from build123d import *

# Parameters (mm, degrees)
F0_W     = 50.8
F0_H     = 50.8
F1_DEPTH = 50.8
F3_DEPTH = 50.801
F7_DEPTH = 50.801
F9_DEPTH = 50.801
F11_R    = 1.5875


with BuildPart() as f1:
    # F0 (on Front) → F1 (new body)
    with BuildSketch(Plane.XZ):
        with Locations((25.4, 25.4)):
            Rectangle(F0_W, F0_H)
    extrude(amount=F1_DEPTH)

    # F2 (on face) → F3 (cut, through all)
    with BuildSketch(Plane.YZ.offset(50.8)):
        with BuildLine():
            Line((0, 27.305), (0, 43.815))
            ThreePointArc((0, 43.815), (-0.9299359697, 41.5699359697), (-3.175, 40.64))
            Line((-3.175, 40.64), (-37.465, 40.64))
            ThreePointArc((-37.465, 40.64), (-39.7100640303, 39.7100640303), (-40.64, 37.465))
            Line((-40.64, 37.465), (-40.64, 33.655))
            ThreePointArc((-40.64, 33.655), (-39.7100640303, 31.4099359697), (-37.465, 30.48))
            Line((-37.465, 30.48), (-3.175, 30.48))
            ThreePointArc((-3.175, 30.48), (-0.9299359697, 29.5500640303), (0, 27.305))
        make_face()
        with BuildLine():
            ThreePointArc((-47.625, 20.32), (-49.8700640303, 21.2499359697), (-50.8, 23.495))
            Line((-50.8, 23.495), (-50.8, 6.985))
            ThreePointArc((-50.8, 6.985), (-49.8700640303, 9.2300640303), (-47.625, 10.16))
            Line((-47.625, 10.16), (-13.335, 10.16))
            ThreePointArc((-13.335, 10.16), (-11.0899359697, 11.0899359697), (-10.16, 13.335))
            Line((-10.16, 13.335), (-10.16, 17.145))
            ThreePointArc((-10.16, 17.145), (-11.0899359697, 19.3900640303), (-13.335, 20.32))
            Line((-13.335, 20.32), (-47.625, 20.32))
        make_face()
        with BuildLine():
            Line((0, 50.8), (-3.175, 50.8))
            ThreePointArc((-3.175, 50.8), (-0.9299359697, 49.8700640303), (0, 47.625))
            Line((0, 47.625), (0, 50.8))
        make_face()
        with BuildLine():
            ThreePointArc((-50.8, 47.625), (-49.8700640303, 49.8700640303), (-47.625, 50.8))
            Line((-47.625, 50.8), (-50.8, 50.8))
            Line((-50.8, 50.8), (-50.8, 47.625))
        make_face()
        with BuildLine():
            Line((0, 0), (0, 3.175))
            ThreePointArc((0, 3.175), (-0.9299359697, 0.9299359697), (-3.175, 0))
            Line((-3.175, 0), (0, 0))
        make_face()
        with BuildLine():
            ThreePointArc((-47.625, 0), (-49.8700640303, 0.9299359697), (-50.8, 3.175))
            Line((-50.8, 3.175), (-50.8, 0))
            Line((-50.8, 0), (-47.625, 0))
        make_face()
    extrude(amount=-F3_DEPTH, mode=Mode.SUBTRACT)

    # F6 (on offset) → F7 (cut, through all)
    with BuildSketch(Plane.XZ.offset(50.8)):
        with BuildLine():
            ThreePointArc((3.175, 40.64), (0.9299359697, 41.5699359697), (0, 43.815))
            Line((0, 43.815), (0, 17.145))
            ThreePointArc((0, 17.145), (0.9299359697, 19.3900640303), (3.175, 20.32))
            Line((3.175, 20.32), (6.985, 20.32))
            ThreePointArc((6.985, 20.32), (9.2300640303, 19.3900640303), (10.16, 17.145))
            Line((10.16, 17.145), (10.16, 13.335))
            ThreePointArc((10.16, 13.335), (11.0899359697, 11.0899359697), (13.335, 10.16))
            Line((13.335, 10.16), (17.145, 10.16))
            ThreePointArc((17.145, 10.16), (19.3900640303, 11.0899359697), (20.32, 13.335))
            Line((20.32, 13.335), (20.32, 37.465))
            ThreePointArc((20.32, 37.465), (19.3900640303, 39.7100640303), (17.145, 40.64))
            Line((17.145, 40.64), (3.175, 40.64))
        make_face()
        with BuildLine():
            Line((50.8, 50.8), (47.625, 50.8))
            ThreePointArc((47.625, 50.8), (49.8700640303, 49.8700640303), (50.8, 47.625))
            Line((50.8, 47.625), (50.8, 50.8))
        make_face()
        with BuildLine():
            Line((50.8, 0), (50.8, 43.815))
            ThreePointArc((50.8, 43.815), (49.8700640303, 41.5699359697), (47.625, 40.64))
            Line((47.625, 40.64), (33.655, 40.64))
            ThreePointArc((33.655, 40.64), (31.4099359697, 39.7100640303), (30.48, 37.465))
            Line((30.48, 37.465), (30.48, 3.175))
            ThreePointArc((30.48, 3.175), (29.5500640303, 0.9299359697), (27.305, 0))
            Line((27.305, 0), (50.8, 0))
        make_face()
        with BuildLine():
            ThreePointArc((3.175, 0), (0.9299359697, 0.9299359697), (0, 3.175))
            Line((0, 3.175), (0, 0))
            Line((0, 0), (3.175, 0))
        make_face()
        with BuildLine():
            Line((0, 50.8), (0, 47.625))
            ThreePointArc((0, 47.625), (0.9299359697, 49.8700640303), (3.175, 50.8))
            Line((3.175, 50.8), (0, 50.8))
        make_face()
    extrude(amount=-F7_DEPTH, mode=Mode.SUBTRACT)

    # F8 (on offset) → F9 (cut, through all)
    with BuildSketch(Plane.XY.offset(50.8)):
        with BuildLine():
            ThreePointArc((3.175, -50.8), (0.9299359697, -49.8700640303), (0, -47.625))
            Line((0, -47.625), (0, -50.8))
            Line((0, -50.8), (3.175, -50.8))
        make_face()
        with BuildLine():
            Line((0, 0), (0, -3.175))
            ThreePointArc((0, -3.175), (0.9299359697, -0.9299359697), (3.175, 0))
            Line((3.175, 0), (0, 0))
        make_face()
        with BuildLine():
            ThreePointArc((50.8, -47.625), (49.8700640303, -49.8700640303), (47.625, -50.8))
            Line((47.625, -50.8), (50.8, -50.8))
            Line((50.8, -50.8), (50.8, -47.625))
        make_face()
        with BuildLine():
            ThreePointArc((17.145, -35.56), (19.3900640303, -34.6300640303), (20.32, -32.385))
            Line((20.32, -32.385), (20.32, -18.415))
            ThreePointArc((20.32, -18.415), (19.3900640303, -16.1699359697), (17.145, -15.24))
            Line((17.145, -15.24), (13.335, -15.24))
            ThreePointArc((13.335, -15.24), (11.0899359697, -16.1699359697), (10.16, -18.415))
            Line((10.16, -18.415), (10.16, -32.385))
            ThreePointArc((10.16, -32.385), (11.0899359697, -34.6300640303), (13.335, -35.56))
            Line((13.335, -35.56), (17.145, -35.56))
        make_face()
        with BuildLine():
            Line((50.8, 0), (27.305, 0))
            ThreePointArc((27.305, 0), (29.5500640303, -0.9299359697), (30.48, -3.175))
            Line((30.48, -3.175), (30.48, -32.385))
            ThreePointArc((30.48, -32.385), (31.4099359697, -34.6300640303), (33.655, -35.56))
            Line((33.655, -35.56), (47.625, -35.56))
            ThreePointArc((47.625, -35.56), (49.8700640303, -36.4899359697), (50.8, -38.735))
            Line((50.8, -38.735), (50.8, 0))
        make_face()
    extrude(amount=-F9_DEPTH, mode=Mode.SUBTRACT)

    # F11 (on offset) → F12 (revolve)
    with BuildSketch(Plane.XZ.offset(25.4)):
        with Locations((25.4, 50.8)):
            Circle(F11_R)
    revolve(axis=Axis((30.3972233087, -25.4, 53.975), (1, 0, 0)))

    # F13 (on face) → F14 (revolve, cut)
    with BuildSketch(Plane.XZ.offset(50.8)):
        with BuildLine():
            Line((23.8125, 47.625), (26.9875, 47.625))
            ThreePointArc((26.9875, 47.625), (25.4, 49.2125), (23.8125, 47.625))
        make_face()
        with BuildLine():
            ThreePointArc((23.8125, 47.625), (25.4, 46.0375), (26.9875, 47.625))
            Line((26.9875, 47.625), (23.8125, 47.625))
        make_face()
    revolve(axis=Axis((27.5035649538, -50.8, 60.325), (1, 0, 0)), mode=Mode.SUBTRACT)


solid = f1.part
CAD build for the part. Positions are in the model's coordinates, mm. A direction names the side the tool comes from. Give positions to 0.01 mm unless a question says otherwise; leave off trailing zeros. Order: outer loops, then holes, each group sorted by start corner. A loop starts at its lowest first (then second) coordinate and runs counter-clockwise, first axis right, second up. Notation, with made-up numbers: (22.5, 62.25) - (79.5, 62.25) arc R21 cw to (79.5, 84.25) - close; hole circle Ø8 at (36.25, 39). An arc over 180 degrees is marked (long way). Answer in a Markdown table with one row per item.
1. Pull direction Z, two halves, no side cores. Call faces 1 (the flat face through (15, -35.56, 46)), 2 (the cylindrical face through (15.44, -0.91, 0.95)), 3 (the cylindrical face through (25.5, -11.1, 19.4)): pulls with the +Z half, pulls with the -Z half, needs draft (parallel to the pull), parting line crosses it, or undercut.
Data:
| item | result |
|---|---|
| face 1 | needs draft |
| face 2 | pulls with the -Z half |
| face 3 | undercut |
2. Saw through at A-A, the plane z = 45. Give the cut face in (x, y) (3 decimals), plus the area to 3 significant figures.
Data:
| item | result |
|---|---|
| outline | (0, -47.625) arc R3.175 ccw to (3.175, -50.8) - (47.625, -50.8) arc R3.175 ccw to (50.8, -47.625) - (50.8, -38.735) arc R3.175 ccw to (47.625, -35.56) - (33.655, -35.56) arc R3.175 cw to (30.48, -32.385) - (30.48, -3.175) arc R3.175 ccw to (27.305, 0) - (3.175, 0) arc R3.175 ccw to (0, -3.175) - close; hole (10.16, -32.385) arc R3.175 ccw to (13.335, -35.56) - (17.145, -35.56) arc R3.175 ccw to (20.32, -32.385) - (20.32, -18.415) arc R3.175 ccw to (17.145, -15.24) - (13.335, -15.24) arc R3.175 ccw to (10.16, -18.415) - close |
| area | 1,650 mm² |
3. Saw through at C-C, the plane y = -31.5. Give the cut face in (x, z) (3 decimals), plus the area to 3 significant figures.
Data:
| item | result |
|---|---|
| outline | (0, 3.175) arc R3.175 ccw to (3.175, 0) - (10.16, 0) - (10.16, 10.16) - (0, 10.16) - close; (0, 43.815) arc R3.175 ccw to (3.175, 40.64) - (10.16, 40.64) - (10.16, 50.8) - (3.175, 50.8) arc R3.175 ccw to (0, 47.625) - close; (20.32, 0) - (27.305, 0) arc R3.175 ccw to (30.48, 3.175) - (30.48, 10.16) - (20.32, 10.16) - close; (20.32, 20.32) - (30.48, 20.32) - (30.48, 30.48) - (20.32, 30.48) - close; (20.32, 40.64) - (30.48, 40.64) - (30.48, 50.8) - (20.32, 50.8) - close |
| area | 507 mm² |
4. Saw through at B-B, the plane x = 4.5. Give the cut face in (y, z) (3 decimals), plus the area to 3 significant figures.
Data:
| item | result |
|---|---|
| outline | (-50.8, 3.175) arc R3.175 ccw to (-47.625, 0) - (-3.175, 0) arc R3.175 ccw to (0, 3.175) - (0, 20.32) - (-13.335, 20.32) arc R3.175 cw to (-10.16, 17.145) - (-10.16, 13.335) arc R3.175 cw to (-13.335, 10.16) - (-47.625, 10.16) arc R3.175 ccw to (-50.8, 6.985) - close; (-50.8, 40.64) - (-3.175, 40.64) arc R3.175 ccw to (0, 43.815) - (0, 47.625) arc R3.175 ccw to (-3.175, 50.8) - (-47.625, 50.8) arc R3.175 ccw to (-50.8, 47.625) - close |
| area | 1,130 mm² |
5. Saw through at D-D, the plane z = 14.5. Give the cut face in (x, y) (3 decimals), plus the area to 3 significant figures.
Data:
| item | result |
|---|---|
| outline | (0, -10.16) - (10.16, -10.16) - (10.16, 0) - (3.175, 0) arc R3.175 ccw to (0, -3.175) - close; (20.32, -10.16) - (30.48, -10.16) - (30.48, -3.175) arc R3.175 ccw to (27.305, 0) - (20.32, 0) - close |
| area | 202 mm² |
6. Tool access for faces 4 (the cylindrical face through (9.21, -5.28, 19.41)), 5 (the flat face through (25, -10.16, 15)), 6 (the flat face through (10.16, -25, 5)), 7 (the cylindrical face through (1, -26.2, 41.5)): list every direction of +Z, -Z, +X, -X, +Y, -Y with a clear straight run to the whole face (end or side of a thin tool).
Data:
| item | result |
|---|---|
| face 4 | +Y, -Y |
| face 5 | +X, -X, -Y |
| face 6 | +Z, -Z |
| face 7 | -X, +Y, -Y |
7. Flat gauge pins, fed straight in: pin 1 (1.9 mm diameter, centred on x = 7, z = 16, fed in from -Y); pin 2 (10 mm diameter, centred on x = 31, y = -44, fed in from +Z); pin 3 (4 mm diameter, centred on x = 25.5, z = 36, fed in from +Y). Where does each tip first touch, or does it go through?
Data:
| item | result |
|---|---|
| pin 1 | stops at y = -10.16 |
| pin 2 | stops at z = 50.8 |
| pin 3 | stops at y = -40.59 |
8. Probe probe 1 along Z at (x, y) = (16.5, -45); probe 2 along Z at (x, y) = (25.5, -9); probe 3 along X at (y, z) = (-6, 46). List the from-to ranges inside material, lowest first. Write a range as [from, to].
Data:
| item | result |
|---|---|
| probe 1 | z = [0, 10.16], [40.64, 50.8] |
| probe 2 | z = [0, 30.48], [40.64, 50.8] |
| probe 3 | x = [0, 30.48] |
